The model under review builds one solid part; all positions refer to its coordinate system, in mm. Face numbers are marked on the shaded views. A direction names the side the tool comes from. Round coordinates to 2 decimals unless told otherwise and drop trailing zeros. Write each loop counter-clockwise with the first axis right and the second up, starting at its lowest first coordinate (ties: lowest second). Pieces come first, ordered by that corner, then holes. Notation, with made-up numbers: (9, 47) -> (66, 47) arc R11 cw to (66, 53) -> close; hole circle Ø9 at (-31.5, 29). An arc over 180 degrees is marked (long way). Answer in a Markdown table with one row per item. Add a question column.
Autodesk Inventor part; units mm, degrees
ref_plane "YZ Plane" through (0, 0, 0) normal (1, 0, 0) x (0, 1, 0)
ref_plane "XZ Plane" through (0, 0, 0) normal (0, 1, 0) x (-1, 0, 0)
ref_plane "XY Plane" through (0, 0, 0) normal (0, 0, 1) x (1, 0, 0)
sketch "Sketch1" plane through (0, 0, 0) normal (0, 0, 1) x (1, 0, 0)
  line L0 (57.5, -32.5) -> (-57.5, -32.5)
  line L1 (-57.5, -32.5) -> (-57.5, 32.5)
  line L2 (-57.5, 32.5) -> (57.5, 32.5)
  line L3 (57.5, 32.5) -> (57.5, -32.5)
  line L4 (50, -25) -> (-50, -25)
  line L5 (-50, -25) -> (-50, 25)
  line L6 (-50, 25) -> (50, 25)
  line L7 (50, 25) -> (50, -25)
  line L8 (57.5, 0) -> (-57.5, 0) construction
  line L9 (0, -32.5) -> (0, 32.5) construction
  line L10 (-37.5, 32.5) -> (-37.5, 25)
  line L11 (-57.5, 17.5) -> (-50, 17.5)
  line L12 (37.5, -25) -> (37.5, -32.5)
  line L13 (50, -17.5) -> (57.5, -17.5)
  line L14 (-37.5, -25) -> (-37.5, -32.5)
  line L15 (-57.5, -17.5) -> (-50, -17.5)
  line L16 (37.5, 32.5) -> (37.5, 25)
  line L17 (50, 17.5) -> (57.5, 17.5)
  line L18 (-53.75, 28.75) -> (53.75, 28.75) construction
  line L19 (53.75, 28.75) -> (53.75, -28.75) construction
  line L20 (53.75, -28.75) -> (-53.75, -28.75) construction
  line L21 (-53.75, -28.75) -> (-53.75, 28.75) construction
  line L22 (-53.75, 28.75) -> (53.75, -28.75) construction
  line L23 (53.75, 28.75) -> (-53.75, -28.75) construction
  point P0 (0, 0)
  point P1 (-35.5, 20)
  point P2 (35.5, 20)
  point P3 (35.5, -20)
  point P4 (-35.5, -20)
  dimension "d0" = 115
  dimension "d1" = 65
  dimension "d2" = 100
  dimension "d3" = 50
  dimension "d4" = 15
  dimension "d5" = 20
  dimension "d6" = 40
  dimension "d7" = 71
extrude "Extrusion1" add sketch "Sketch1" against normal blind 40 contours L0 L12 L4 L7 L13 L3 | L0 L1 L15 L5 L4 L14 | L17 L7 L6 L16 L2 L3 | L1 L2 L10 L6 L5 L11
extrude "Extrusion2" add sketch "Sketch1" along normal blind 10
hole "Hole1" at (-35.5, 20, 0) at (35.5, 20, 0) at (35.5, -20, 0) at (-35.5, -20, 0) direction (0, 0, 1) diameter 3.2 end through all counterbore diameter 6 counterbore depth 5
extrude "Extrusion8" add sketch "Sketch1" against normal blind 40 contours L0 L14 L4 L12 | L13 L7 L17 L3 | L1 L11 L5 L15 | L16 L6 L10 L2
equation "\"epsilon\" = 0"
properties part number "magnet_holder" material "PC/ABS Plastic"
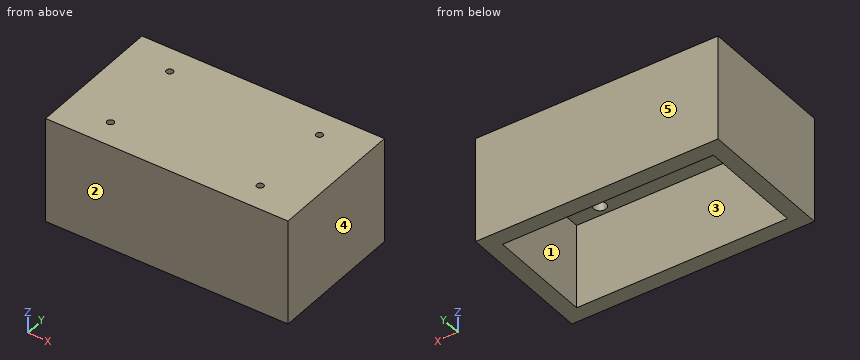
1. Add section C-C on x = 16.5. Write out the cut boundary in (y, z), plus the area to 3 significant figures.
2. For L1, parallel to X at y = -20, z = 2.45; L2, parallel to Y at x = 35.5, z = 3.15; L3, parallel to X at y = 20, z = 6.85, list the stretches that pass through material, from the lowest coordinate up.
3. Insertion check: pin 1 Ø5 at (x, y) = (-35, 19) entering from -Z; pin 2 Ø5 at (x, y) = (-35.5, 20) entering from +Z; pin 3 Ø1.8 at (x, y) = (34.5, -20.5) entering from -Z. Each pin has a flat end and moves straight along its axis. Give the tip position at first contact, or say it passes through.
4. Add section D-D on z = -22. Write out the cut boundary in (x, y).
5. Add section B-B on z = 3. Write out the cut boundary in (x, y).
6. Tool access review of the marked faces 1 and 2: name each direction out of +Z, -Z, +X, -X, +Y, -Y from which nothing blocks a thin tool from reaching the whole face with its end or side.
7. Mouldability with a two-part tool opening along Y and no side actions: class the marked faces 3, 4 and 5 as pulls with the +Y half, pulls with the -Y half, needs draft (parallel to the pull), parting line crosses it, or undercut.
8. Add section A-A on y = -20. Write out the cut boundary in (x, z), plus the area to 3 significant figures.
Filled in:
| question | item | result |
|---|---|---|
| 1 | outline | (-32.5, -40) -> (-25, -40) -> (-25, 0) -> (25, 0) -> (25, -40) -> (32.5, -40) -> (32.5, 10) -> (-32.5, 10) -> close |
| 1 | area | 1,250 mm² |
| 2 | L1 | -57.5 to -38.5, -32.5 to 32.5, 38.5 to 57.5 |
| 2 | L2 | -32.5 to -23, -17 to 17, 23 to 32.5 |
| 2 | L3 | -57.5 to -37.1, -33.9 to 33.9, 37.1 to 57.5 |
| 3 | pin 1 | z = 0 |
| 3 | pin 2 | z = 10 |
| 3 | pin 3 | z = 5 |
| 4 | outline | (-57.5, -32.5) -> (57.5, -32.5) -> (57.5, 32.5) -> (-57.5, 32.5) -> close; hole (-50, -25) -> (50, -25) -> (50, 25) -> (-50, 25) -> close |
| 5 | outline | (-57.5, -32.5) -> (57.5, -32.5) -> (57.5, 32.5) -> (-57.5, 32.5) -> close; hole circle Ø6 at (-35.5, -20); hole circle Ø6 at (-35.5, 20); hole circle Ø6 at (35.5, -20); hole circle Ø6 at (35.5, 20) |
| 6 | face 1 | -Z |
| 6 | face 2 | +Z, -Z, +X, -X, -Y |
| 7 | face 3 | undercut |
| 7 | face 4 | needs draft |
| 7 | face 5 | pulls with the +Y half |
| 8 | outline | (-57.5, -40) -> (-50, -40) -> (-50, 0) -> (-38.5, 0) -> (-38.5, 5) -> (-37.1, 5) -> (-37.1, 10) -> (-57.5, 10) -> close; (-33.9, 5) -> (-32.5, 5) -> (-32.5, 0) -> (32.5, 0) -> (32.5, 5) -> (33.9, 5) -> (33.9, 10) -> (-33.9, 10) -> close; (37.1, 5) -> (38.5, 5) -> (38.5, 0) -> (50, 0) -> (50, -40) -> (57.5, -40) -> (57.5, 10) -> (37.1, 10) -> close |
| 8 | area | 1,660 mm² |
